Here's how the part is built. I have some questions about the finished solid (model axes, mm). Face numbers are marked on the shaded views. A direction names the side the tool comes from. Coordinates: 2 decimals unless noted, no trailing zeros. Write each loop counter-clockwise with the first axis right and the second up, starting at its lowest first coordinate (ties: lowest second). Pieces come first, ordered by that corner, then holes. Notation, with made-up numbers: (38, 80.25) -> (44, 80.25) arc R11 cw to (44, 94.25) -> close; hole circle Ø11 at (-33.75, 65.5). An arc over 180 degrees is marked (long way). Use a Markdown table: item, result. Add a question column.
Item 1: Imagine slicing it at B-B, the plane y = 8.5. Write out the boundary of the cut face in (x, z), and give its area (3 significant figures).
Item 2: On a 3-axis mill with a long thin cutter (end or side, diameter ignored), from which of +Z, -Z, +X, -X, +Y, -Y can I reach the whole of each face in a straight line? I mean the marked faces 1 and 2. Say none if no direction works.
Item 3: Will these pins go through, and if not, where does the flat tip stop? pin 1 Ø12 at (y, z) = (9.5, -23) entering from +X; pin 2 Ø1 at (x, y) = (-26, 23) entering from +Z; pin 3 Ø10 at (y, z) = (10, -13.5) entering from -X.
Item 4: If I drill on line 1 along Y through (x, z) = (39, -0.7); line 2 along Z through (x, y) = (1, 23.75); line 3 along Z through (x, y) = (-32, 26), over which ranges is the centre line in solid material (lowest first)? Write a range as from..to.
Item 5: Imagine slicing it at A-A, the plane x = 12. Write out the boundary of the cut face in (y, z).
Item 6: Imagine slicing it at C-C, the plane y = 17. Write out the boundary of the cut face in (x, z), and give its area (3 significant figures).
Item 7: Imagine slicing it at D-D, the plane y = 2.5. Write out the boundary of the cut face in (x, z), and give its area (3 significant figures).
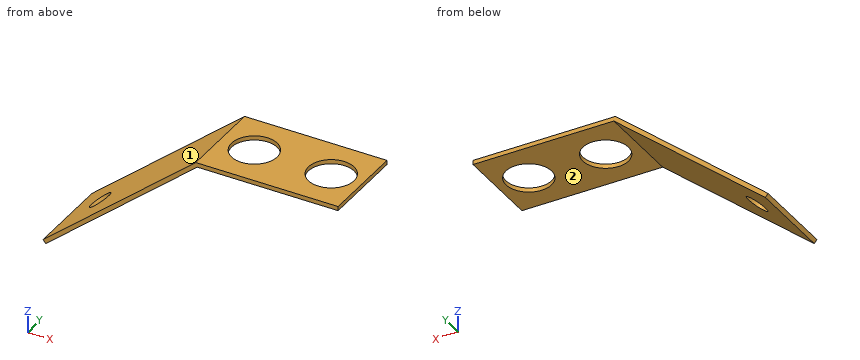
```python
from build123d import *

# Parameters (mm, degrees)
EXTRUDE_THIN1_DEPTH = 30
SKETCH2_R           = 4
CUT_EXTRUDE1_DEPTH  = 10
SKETCH3_R           = 8
CUT_EXTRUDE2_DEPTH  = 10


with BuildPart() as part:
    # Sketch1 → Extrude-Thin1 (new body)
    with BuildSketch(Plane(origin=(0, 0, 0), x_dir=(1, 0, 0), z_dir=(0, 1, 0))):
        Polygon((-53.623111018, 44.995132678), (0, 0), (50, 0), (50, 1.5), (0.545955351, 1.5), (-52.658929604, 46.144199343), align=None)
    extrude(amount=EXTRUDE_THIN1_DEPTH)

    # Sketch2 → Cut-Extrude1 (cut)
    with BuildSketch(Plane(origin=(0, 0, 0), x_dir=(0.7660444431189818, 0, 0.6427876096865349), z_dir=(-0.6427876096865348, 0, 0.7660444431189817))):
        with Locations((-55, 15)):
            Circle(SKETCH2_R)
    extrude(amount=-CUT_EXTRUDE1_DEPTH, mode=Mode.SUBTRACT)

    # Sketch3 → Cut-Extrude2 (cut)
    with BuildSketch(Plane.XY):
        with Locations((12, 15)):
            Circle(SKETCH3_R)
        with Locations((39, 15)):
            Circle(SKETCH3_R)
    extrude(amount=-CUT_EXTRUDE2_DEPTH, mode=Mode.SUBTRACT)


solid = part.part
```
Ans:
| question | item | result |
|---|---|---|
| 1 | outline | (-53.62, -45) -> (-52.66, -46.14) -> (0.55, -1.5) -> (7.34, -1.5) -> (7.34, 0) -> (0, 0) -> close; (16.66, -1.5) -> (34.34, -1.5) -> (34.34, 0) -> (16.66, 0) -> close; (43.66, -1.5) -> (50, -1.5) -> (50, 0) -> (43.66, 0) -> close |
| 1 | area | 151 mm^2 |
| 2 | face 1 | +Z, -X, +Y, -Y |
| 2 | face 2 | -Z, +X, +Y, -Y |
| 3 | pin 1 | stops at x = -17.93 |
| 3 | pin 2 | stops at z = -21.4 |
| 3 | pin 3 | stops at x = -22.05 |
| 4 | line 1 | y = 0..7, 23..30 |
| 4 | line 2 | z = -1.5..0 |
| 4 | line 3 | z = -28.81..-26.85 |
| 5 | outline | (0, -1.5) -> (7, -1.5) -> (7, 0) -> (0, 0) -> close; (23, -1.5) -> (30, -1.5) -> (30, 0) -> (23, 0) -> close |
| 6 | outline | (-53.62, -45) -> (-52.66, -46.14) -> (-43.82, -38.73) -> (-44.79, -37.58) -> close; (-39.48, -33.13) -> (-38.51, -34.28) -> (0.55, -1.5) -> (4.25, -1.5) -> (4.25, 0) -> (0, 0) -> close; (19.75, -1.5) -> (31.25, -1.5) -> (31.25, 0) -> (19.75, 0) -> close; (46.75, -1.5) -> (50, -1.5) -> (50, 0) -> (46.75, 0) -> close |
| 6 | area | 122 mm^2 |
| 7 | outline | (-53.62, -45) -> (-52.66, -46.14) -> (0.55, -1.5) -> (50, -1.5) -> (50, 0) -> (0, 0) -> close |
| 7 | area | 179 mm^2 |
